The model under review builds one solid part; all positions refer to its coordinate system, in mm. Face numbers are marked on the shaded views. Round coordinates to 2 decimals unless told otherwise and drop trailing zeros. Loops run counter-clockwise (first coordinate to the right, second up) from the corner with the lowest first, then second, coordinate; pieces in that order, holes last. Notation, with made-up numbers: M 49,87.25 L 72,87.25 A7 cw 72,93.25 Z; hole C 17.25,45.5 d7. An arc over 180 degrees is marked long. One line per question, with ' | ' between items.
Autodesk Inventor part; units mm, degrees
ref_plane "NUT_ROD_XY" through (0, 0, 0) normal (1, 0, 0) x (0, 0, -1)
ref_plane "NUT_ROD_YZ" through (0, 0, 0) normal (0, 0, -1) x (0, 1, 0)
ref_plane "NUT_ROD_ZX" through (0, 0, 0) normal (0, 1, 0) x (1, 0, 0)
sketch "Sketch_1" plane through (0, 0, 0) normal (0, 0, 1) x (1, 0, 0)
  line L0 (3, 0) -> (-3, 0)
  line L1 (-3, 8.5) -> (-3, 5)
  line L2 (-3, 5) -> (-2.3235, 4.3235)
  line L3 (-2.3235, 4.3235) -> (2.3235, 4.3235)
  line L4 (2.3235, 4.3235) -> (3, 5)
  line L5 (3, 5) -> (3, 8.5)
  line L6 (3, 8.5) -> (1.6335, 13.6)
  line L7 (1.6335, 13.6) -> (-1.6335, 13.6)
  line L8 (-1.6335, 13.6) -> (-3, 8.5)
revolve "Revolution1" add sketch "Sketch_1" angle 360 about axis through (3, 0, 0) along (1, 0, 0)
thread "Thread1"
sketch "Sketch_2" plane through (0, 0, 0) normal (1, 0, 0) x (0, 1, 0)
  circle A0 centre (0, 0) radius 17
  line L0 (-4.9075, 8.5) -> (-9.815, 0)
  line L1 (-9.815, 0) -> (-4.9075, -8.5)
  line L2 (-4.9075, -8.5) -> (4.9075, -8.5)
  line L3 (4.9075, -8.5) -> (9.815, 0)
  line L4 (9.815, 0) -> (4.9075, 8.5)
  line L5 (4.9075, 8.5) -> (-4.9075, 8.5)
extrude "Extrusion1" cut sketch "Sketch_2" along normal mid plane 12
ref_plane "NUT_ROD_XY" through (0, 0, 0) normal (1, 0, 0) x (0, 0, -1)
ref_plane "NUT_ROD_YZ" through (0, 0, 0) normal (0, 0, -1) x (0, 1, 0)
ref_plane "NUT_ROD_ZX" through (0, 0, 0) normal (0, 1, 0) x (1, 0, 0)
properties part number "NT-03_CQS"
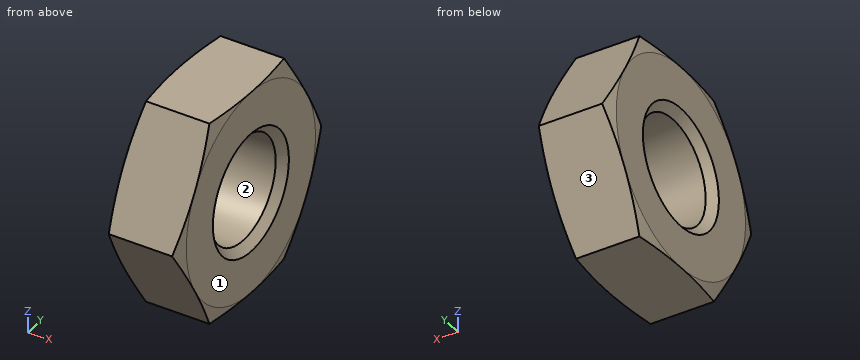
1) For line 1 (Z direction, x = -0.55, y = 0); line 2 (Z direction, x = 1.25, y = -1); line 3 (Y direction, x = 1.45, z = 1.5), list the stretches that pass through material, from the lowest coordinate up.
Output values:
line 1: z = -8.5 to -4.32, 4.32 to 8.5 | line 2: z = -8.5 to -4.21, 4.21 to 8.5 | line 3: y = -8.95 to -4.05, 4.05 to 8.95
2) Mouldability with a two-part tool opening along Y and no side actions: class the marked faces 1, 2 and 3 as +Y half, -Y half, draft (parallel to the pull), parting line (faces both ways), or undercut.
Output values:
face 1: draft | face 2: undercut | face 3: +Y half
3) Add section A-A on x = -0.1. State the section outline as (y, z) points (1 decimal).
Output values:
outline: M -9.8,0 L -4.9,-8.5 L 4.9,-8.5 L 9.8,0 L 4.9,8.5 L -4.9,8.5 Z; hole C 0,0 d8.6
